Job drawing, mm, ordinate dimensions from the low corner. One solid piece. A direction names the side the tool comes from. Coordinates: 2 decimals unless noted, no trailing zeros. Order: outer loops, then holes, each group sorted by start corner. A loop starts at its lowest first (then second) coordinate and runs counter-clockwise, first axis right, second up. Notation, with made-up numbers: (69, -3.5) -> (73, -3.5) arc R19 ccw to (73, 10.5) -> close; hole circle Ø10 at (6, 30). An arc over 180 degrees is marked (long way). Use CSV: the item, a comma, the result in double quotes. Start each with the question number.
(1) Tool access for the marked faces 1 and 2: list every direction of +Z, -Z, +X, -X, +Y, -Y with a clear straight run to the whole face (end or side of a thin tool).
(2) Cut at D-D on x = 6. Write the cut outline in (y, z) (1 decimal).
(3) Cut at A-A on x = 30. Write the cut outline in (y, z) (1 decimal).
(4) Cut at C-C on z = 4.2. Write the cut outline in (x, y), plus the area to 3 significant figures.
(5) Cut at B-B on y = 15. Write the cut outline in (x, z) (1 decimal).
(6) Pull direction X, two halves, no side cores. Call the marked faces 3 and 4: pulls with the +X half, pulls with the -X half, needs draft (parallel to the pull), parting line crosses it, or undercut.
(7) Probe L1, parallel to Y at x = 39.5, z = 1.85; L2, parallel to Y at x = 30, z = 2.1 (1 decimal); L3, parallel to Y at x = 30, z = 0.8. List the from-to ranges inside material, lowest first.
(8) Pin check, flat tips, straight feed: pin 1 Ø5 at (x, y) = (32, 27) entering from -Z (3 decimals); pin 2 Ø1.2 at (x, z) = (31, 2.5) entering from +Y; pin 3 Ø10 at (x, y) = (52, 15) entering from -Z (3 decimals). Stop position of each tip, or through.
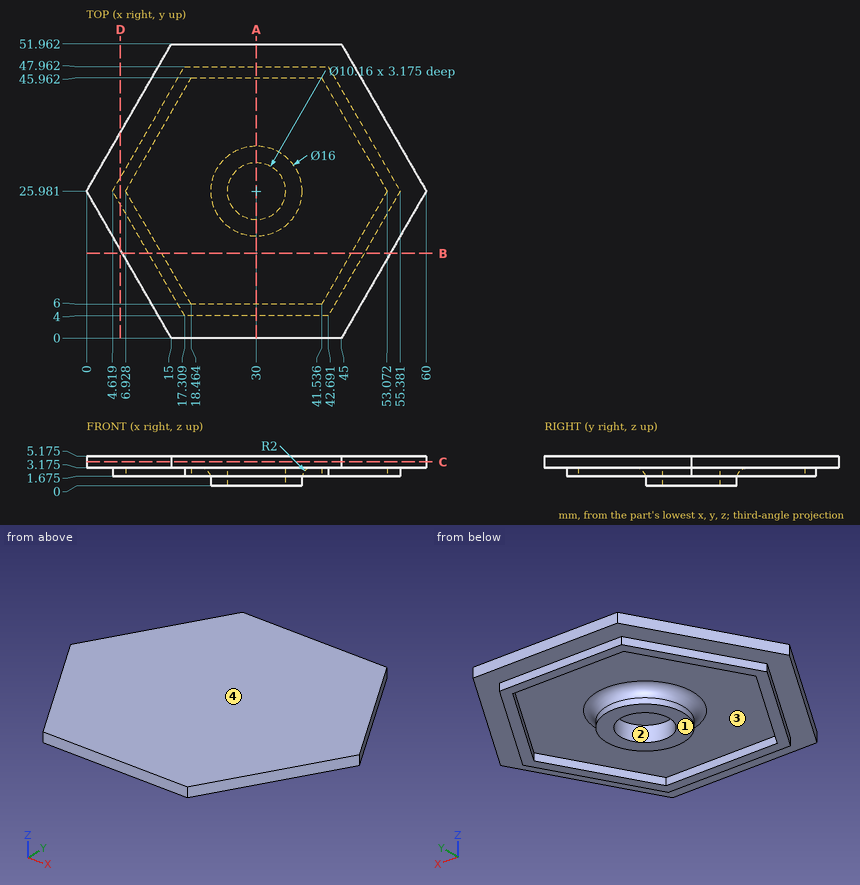
Outcome:
1,face 1,"-Z, +X, -X, +Y, -Y"
1,face 2,"-Z"
2,outline,"(15.6, 3.2) -> (23.6, 3.2) -> (23.6, 1.7) -> (28.4, 1.7) -> (28.4, 3.2) -> (36.4, 3.2) -> (36.4, 5.2) -> (15.6, 5.2) -> close"
3,outline,"(0, 3.2) -> (4, 3.2) -> (4, 1.7) -> (6, 1.7) -> (6, 3.2) -> (16, 3.2) arc R2 cw to (18, 1.2) -> (18, 0) -> (20.9, 0) -> (20.9, 3.2) -> (31.1, 3.2) -> (31.1, 0) -> (34, 0) -> (34, 1.2) arc R2 cw to (36, 3.2) -> (46, 3.2) -> (46, 1.7) -> (48, 1.7) -> (48, 3.2) -> (52, 3.2) -> (52, 5.2) -> (0, 5.2) -> close"
4,outline,"(0, 25.98) -> (15, 0) -> (45, 0) -> (60, 25.98) -> (45, 51.96) -> (15, 51.96) -> close"
4,area,"2,340 mm2"
5,outline,"(6.3, 3.2) -> (11, 3.2) -> (11, 1.7) -> (13.3, 1.7) -> (13.3, 3.2) -> (46.7, 3.2) -> (46.7, 1.7) -> (49, 1.7) -> (49, 3.2) -> (53.7, 3.2) -> (53.7, 5.2) -> (6.3, 5.2) -> close"
6,face 3,"undercut"
6,face 4,"needs draft"
7,L1,"4 to 6, 45.96 to 47.96"
7,L2,"4 to 6, 17.8 to 20.9, 31.1 to 34.2, 46 to 48"
7,L3,"17.98 to 20.9, 31.06 to 33.98"
8,pin 1,"z = 3.175"
8,pin 2,"y = 47.96"
8,pin 3,"z = 1.675"
